For this review, take the finished solid that the model builds, in its own axes (mm). Coordinates: 2 decimals unless noted, no trailing zeros. Loops run counter-clockwise (first coordinate to the right, second up) from the corner with the lowest first, then second, coordinate; pieces in that order, holes last. Notation, with made-up numbers: M 13,66.5 L 67,66.5 A14 cw 67,75.5 Z; hole C 6.25,45.25 d1. An arc over 180 degrees is marked long. Answer as a JSON object with one key per item and string values. Group by question number.
Item 1: Insertion check: pin 1 (1.5 mm diameter, centred on x = 2.5, z = 1, fed in from +Y); pin 2 (1.4 mm diameter, centred on x = 1.59, y = 2.38, fed in from -Z). Each pin has a flat end and moves straight along its axis. Give the tip position at first contact, or say it passes through.
Item 2: Add section C-C (z = 3). State the section outline as (x, y) points (1 decimal), then the cut area to 3 significant figures.
Item 3: Add section B-B (y = 3). State the section outline as (x, z) points, then the cut area to 3 significant figures.
Item 4: Wall thickness on L1, parallel to X at y = 2.5, z = 3.25; L2, parallel to Y at x = 1.55, z = -0.25; L3, parallel to Z at x = 1.5, y = -2: over which ranges is each line inside the solid? List them lowest first. Write a range as from..to.
Item 5: Add section D-D (x = 2.9). State the section outline as (y, z) points.
Item 6: Mouldability with a two-part tool opening along Y and no side actions: class faces 1 (the face through (2, -2.381, 0)), 2 (the face through (1.002, 2.918, 0.056)), 3 (the face through (0, 0, 0)) as +Y half, -Y half, draft (parallel to the pull), parting line (faces both ways), or undercut.
Item 7: Add section A-A (x = 1.8). State the section outline as (y, z) points.
from build123d import *

# Parameters (mm, degrees)
F0_W     = 4.7625
F0_H     = 4.7625
F1_DEPTH = 3.175
F2_R     = 1.5875
F3_DEPTH = 6.35
F4_DEPTH = 1.5875
F5_R     = 0.79375
F6_DEPTH = 7.9385


with BuildPart() as f1:
    # F0 (on Right) → F1 (new body)
    with BuildSketch(Plane.YZ):
        Rectangle(F0_W, F0_H)
    extrude(amount=F1_DEPTH)

    # F2 (on face) → F3 (join)
    with BuildSketch(Plane.XY.offset(2.38125)):
        with Locations((1.5875, 2.38125)):
            Circle(F2_R)
    extrude(amount=-F3_DEPTH)

    # F2 (on face) → F4 (join)
    with BuildSketch(Plane.XY.offset(2.38125)):
        with Locations((1.5875, 2.38125)):
            Circle(F2_R)
    extrude(amount=F4_DEPTH)

    # F5 (on face) → F6 (cut, through all)
    with BuildSketch(Plane.XY.offset(3.96875)):
        with Locations((1.5875, 2.38125)):
            Circle(F5_R)
    extrude(amount=-F6_DEPTH, mode=Mode.SUBTRACT)


solid = f1.part
From the geometry:
{
 "1": {"pin 1": "stops at y = 3.96", "pin 2": "passes through"},
 "2": {"outline": "C 1.6,2.4 d3.2; hole C 1.6,2.4 d1.6", "area": "5.94 mm²"},
 "3": {"outline": "M 0.13,-3.97 L 1.09,-3.97 L 1.09,3.97 L 0.13,3.97 Z; M 2.08,-3.97 L 3.05,-3.97 L 3.05,3.97 L 2.08,3.97 Z", "area": "15.3 mm²"},
 "4": {"L1": "x = 0..0.8, 2.37..3.17", "L2": "y = -2.38..1.59, 3.17..3.97", "L3": "z = -2.38..2.38"},
 "5": {"outline": "M -2.38,-2.38 L 1.49,-2.38 L 1.49,-3.97 L 3.27,-3.97 L 3.27,3.97 L 1.49,3.97 L 1.49,2.38 L -2.38,2.38 Z"},
 "6": {"face 1": "-Y half", "face 2": "undercut", "face 3": "draft"},
 "7": {"outline": "M -2.38,-2.38 L 0.81,-2.38 L 0.81,-3.97 L 1.62,-3.97 L 1.62,3.97 L 0.81,3.97 L 0.81,2.38 L -2.38,2.38 Z; M 3.15,-3.97 L 3.95,-3.97 L 3.95,3.97 L 3.15,3.97 Z"}
}
